Can you work these out from the model? Positions are in its coordinate system, mm. Coordinates: 2 decimals unless noted, no trailing zeros. Order: outer loops, then holes, each group sorted by start corner. A loop starts at its lowest first (then second) coordinate and runs counter-clockwise, first axis right, second up. Notation, with made-up numbers: (1.5, 87) - (53.5, 87) arc R18 cw to (53.5, 119) - close; hole circle Ø8 at (12, 52.25). An arc over 180 degrees is marked (long way). Use a Markdown table: item, result. Add a question column.
(1) I want a section at A-A (y = 1.1). State how many separate pieces and enclosed holes the cut face has, and give its area (3 significant figures).
(2) I want a section at C-C (z = -7). List the corners of the cut face in (x, y) for me (3 decimals), and give its area (3 significant figures).
(3) If I drill on L1, parallel to Z at x = 222.5, y = 1.7; L2, parallel to Z at x = -87, y = 0.85; L3, parallel to X at y = 0.6, z = 109.5, over which ranges is the centre line in solid material (lowest first)? Write a range as [from, to].
(4) For pin 1 Ø4.5 at (x, z) = (152.4, -69.68) entering from +Y; pin 2 Ø1 at (y, z) = (1, 96) entering from +X, each with a flat end and sliding along its axis, tell me the tip position at first contact or that it passes through.
(5) I want a section at B-B (x = 261.5). List the corners of the cut face in (y, z) for me (3 decimals).
```python
from build123d import *

# Parameters (mm, degrees)
SKETCH1_W           = 304.8
SKETCH1_H           = 508
BOSS_EXTRUDE1_DEPTH = 3.175
SKETCH4_W           = 254.003143871
SKETCH4_H           = 3.175
BOSS_EXTRUDE2_DEPTH = 152.4
FILLET1_R           = 25.4
FILLET2_R           = 25.4
SKETCH2_R           = 2.38125
CUT_EXTRUDE3_DEPTH  = 152.4
FILLET3_R           = 25.4
SKETCH5_R           = 2.38125
CUT_EXTRUDE4_DEPTH  = 397.775399592


with BuildPart() as part:
    # Sketch1 → Boss-Extrude1 (new body)
    with BuildSketch(Plane(origin=(0, 0, 0), x_dir=(1, 0, 0), z_dir=(0, 1, 0))):
        Rectangle(SKETCH1_W, SKETCH1_H)
    extrude(amount=BOSS_EXTRUDE1_DEPTH)

    # Sketch4 → Boss-Extrude2 (add)
    with BuildSketch(Plane(origin=(152.4, 0, 0), x_dir=(0, 0, -1), z_dir=(1, 0, 0))):
        with Locations((127.001571936, 1.5875)):
            Rectangle(SKETCH4_W, SKETCH4_H)
    extrude(amount=BOSS_EXTRUDE2_DEPTH)

    # Fillet1
    fillet1_edges = [part.edges().sort_by_distance(p)[0] for p in [
        (152.4, 1.5875, 0),
    ]]
    fillet(fillet1_edges, radius=FILLET1_R)

    # Fillet2
    fillet2_edges = [part.edges().sort_by_distance(p)[0] for p in [
        (304.8, 1.5875, -254.003143871),
        (304.8, 1.5875, 0),
    ]]
    fillet(fillet2_edges, radius=FILLET2_R)

    # Sketch2 → Cut-Extrude3 (cut)
    with BuildSketch(Plane(origin=(0, 3.175, 0), x_dir=(1, 0, 0), z_dir=(0, 1, 0))):
        with Locations(Location((139.7, -127.172447344, 0), (0, 0, 270))):
            Circle(SKETCH2_R)
        with Locations(Location((139.7, 114.127552656, 0), (0, 0, 270))):
            Circle(SKETCH2_R)
    extrude(amount=-CUT_EXTRUDE3_DEPTH, mode=Mode.SUBTRACT)

    # Fillet3
    fillet3_edges = [part.edges().sort_by_distance(p)[0] for p in [
        (152.4, 1.5875, 254),
    ]]
    fillet(fillet3_edges, radius=FILLET3_R)

    # Sketch5 → Cut-Extrude4 (cut, through all)
    with BuildSketch(Plane(origin=(0, 3.175, 0), x_dir=(1, 0, 0), z_dir=(0, 1, 0))):
        with Locations(Location((152.4, 69.677552656, 0), (0, 0, 270))):
            Circle(SKETCH5_R)
        with Locations(Location((222.25, 95.077552656, 0), (0, 0, 270))):
            Circle(SKETCH5_R)
        with Locations(Location((139.7, 114.127552656, 0), (0, 0, 270))):
            Circle(SKETCH5_R)
    extrude(amount=-CUT_EXTRUDE4_DEPTH, mode=Mode.SUBTRACT)


solid = part.part
```
Answers follow:
| question | item | result |
|---|---|---|
| 1 | separate pieces | 1 |
| 1 | enclosed holes | 4 |
| 1 | area | 193,000 mm² |
| 2 | outline | (-152.4, 0) - (296.91, 0) - (296.91, 3.175) - (-152.4, 3.175) - close |
| 2 | area | 1,430 mm² |
| 3 | L1 | z = [-254, -97.45], [-92.71, 0] |
| 3 | L2 | z = [-254, 254] |
| 3 | L3 | x = [-152.4, 152.4] |
| 4 | pin 1 | passes through |
| 4 | pin 2 | stops at x = 152.4 |
| 5 | outline | (0, -254.003) - (3.175, -254.003) - (3.175, 0) - (0, 0) - close |
